Build history of the part. All positions in model axes, mm. A direction names the side the tool comes from. Coordinates: 2 decimals unless noted, no trailing zeros. Loops run counter-clockwise (first coordinate to the right, second up) from the corner with the lowest first, then second, coordinate; pieces in that order, holes last. Notation, with made-up numbers: (14.5, 17.25) - (21.5, 17.25) arc R16 cw to (21.5, 21.25) - close; hole circle Ø6 at (68.25, 7.5). An arc over 180 degrees is marked (long way). One line per item, written item: value.
```python
from build123d import *

# Parameters (mm, degrees)
ESQUISSE1_R             = 18.4
BOSS_EXTRU_1_DEPTH      = 1.5
ESQUISSE3_R             = 1.5
ENL_V_MAT_EXTRU_1_DEPTH = 10
ESQUISSE4_W             = 2.4
ESQUISSE4_H             = 12.5
BOSS_EXTRU_2_DEPTH      = 10
ESQUISSE5_R             = 2.4
BOSS_EXTRU_3_DEPTH      = 8
CONG_1_R                = 1


with BuildPart() as part:
    # Esquisse1 → Boss.-Extru.1 (new body)
    with BuildSketch(Plane.XY):
        Circle(ESQUISSE1_R)
    extrude(amount=BOSS_EXTRU_1_DEPTH)

    # Esquisse3 → Enlèv. mat.-Extru.1 (cut)
    with BuildSketch(Plane(origin=(0, 0, 0), x_dir=(-1, 0, 0), z_dir=(0, 0, -1))):
        with Locations((28.033142688, 46.078269557)):
            Circle(ESQUISSE3_R)
        with Locations((28.033142688, 24.878269557)):
            Circle(ESQUISSE3_R)
        with Locations((5.933142688, 24.878269557)):
            Circle(ESQUISSE3_R)
        with Locations((5.933142688, 46.078269557)):
            Circle(ESQUISSE3_R)
        with Locations((11.130946107, 10.522350341)):
            Circle(ESQUISSE3_R)
        with Locations((11.130946107, -10.677649659)):
            Circle(ESQUISSE3_R)
        with Locations((-10.969053893, -10.677649659)):
            Circle(ESQUISSE3_R)
        with Locations((-10.969053893, 10.522350341)):
            Circle(ESQUISSE3_R)
    extrude(amount=-ENL_V_MAT_EXTRU_1_DEPTH, mode=Mode.SUBTRACT)

    # Esquisse4 → Boss.-Extru.2 (add)
    with BuildSketch(Plane(origin=(0, 0, 0), x_dir=(-1, 0, 0), z_dir=(0, 0, -1))):
        with Locations((13.95, 0)):
            Rectangle(ESQUISSE4_W, ESQUISSE4_H)
        with Locations((-13.95, 0)):
            Rectangle(ESQUISSE4_W, ESQUISSE4_H)
    extrude(amount=BOSS_EXTRU_2_DEPTH)

    # Esquisse5 → Boss.-Extru.3 (add)
    with BuildSketch(Plane.XY.offset(1.5)):
        with Locations((6, 5.7)):
            Circle(ESQUISSE5_R)
        with Locations((6, -5.7)):
            Circle(ESQUISSE5_R)
        with Locations((-6, -5.7)):
            Circle(ESQUISSE5_R)
        with Locations((-6, 5.7)):
            Circle(ESQUISSE5_R)
    extrude(amount=BOSS_EXTRU_3_DEPTH)

    # Congé1
    cong_1_edges = [part.edges().sort_by_distance(p)[0] for p in [
        (3.6, 5.7, 9.5),
        (3.6, -5.7, 9.5),
        (-8.4, -5.7, 9.5),
        (-8.4, 5.7, 9.5),
    ]]
    fillet(cong_1_edges, radius=CONG_1_R)


solid = part.part
```
Item 1: Probe probe 1 along Z at (x, y) = (-2, -11); probe 2 along Y at (x, z) = (10.5, 0.5); probe 3 along X at (y, z) = (-3.5, 4.5). List the from-to ranges inside material, lowest first. Write a range as from..to.
Check result:
probe 1: z = 0..1.5
probe 2: y = -15.11..-12.1, -9.25..9.1, 11.95..15.11
probe 3: x = -6.96..-5.04, 5.04..6.96
Item 2: Pull direction Y, two halves, no side cores. Call faces 5 (the face through (-12.75, 0, -5)), 6 (the face through (-14, -6.25, -5)), 7 (the face through (4.23, -4.08, 4.95)): released by +Y, released by -Y, zero draft, split by the parting line, or undercut.
Check result:
face 5: zero draft
face 6: released by -Y
face 7: undercut
Item 3: Drop flat-ended pins along their axis: P1, Ø2.5, axis at x = -14, z = -4, coming from the +Y side; P2, Ø8, axis at y = 2, z = -6.5, coming from the -X side; P3, Ø3, axis at x = -11, z = 0.5, coming from the +Y side. Give the stop position or say it passes through.
Check result:
P1: stops at y = 6.25
P2: stops at x = -15.15
P3: stops at y = 15.76
Item 4: Tool access for faces 1 (the face through (0, 0, 1.5)), 2 (the face through (-14, 6.25, -5)), 3 (the face through (-15.15, 0, -5)), 4 (the face through (14, -6.25, -5)): list every direction of +Z, -Z, +X, -X, +Y, -Y with a clear straight run to the whole face (end or side of a thin tool).
Check result:
face 1: +Z
face 2: -Z, +X, -X, +Y
face 3: -Z, -X, +Y, -Y
face 4: -Z, +X, -X, -Y
Item 5: Cut at A-A, the plane y = 0. Write the cut outline in (x, z).
Check result:
outline: (-18.4, 0) - (-15.15, 0) - (-15.15, -10) - (-12.75, -10) - (-12.75, 0) - (12.75, 0) - (12.75, -10) - (15.15, -10) - (15.15, 0) - (18.4, 0) - (18.4, 1.5) - (-18.4, 1.5) - close
Item 6: Cut at D-D, the plane y = 10. Write the cut outline in (x, z), then the cut area to 3 significant figures.
Check result:
outline: (-15.45, 0) - (-12.54, 0) - (-12.54, 1.5) - (-15.45, 1.5) - close; (-9.72, 0) - (9.56, 0) - (9.56, 1.5) - (-9.72, 1.5) - close; (12.38, 0) - (15.45, 0) - (15.45, 1.5) - (12.38, 1.5) - close
area: 37.9 mm^2
Item 7: Cut at B-B, the plane x = 11. Write the cut outline in (y, z), then the cut area to 3 significant figures.
Check result:
outline: (-14.75, 0) - (-12.18, 0) - (-12.18, 1.5) - (-14.75, 1.5) - close; (-9.18, 0) - (9.02, 0) - (9.02, 1.5) - (-9.18, 1.5) - close; (12.02, 0) - (14.75, 0) - (14.75, 1.5) - (12.02, 1.5) - close
area: 35.3 mm^2
Item 8: Cut at C-C, the plane z = 0.75. Write the cut outline in (x, y), then the cut area to 3 significant figures.
Check result:
outline: circle Ø36.8 at (0, 0); hole circle Ø3 at (-11.13, -10.68); hole circle Ø3 at (-11.13, 10.52); hole circle Ø3 at (10.97, -10.68); hole circle Ø3 at (10.97, 10.52)
area: 1,040 mm^2
